Could you check a few things on this model? Use its own coordinates, in mm. Face numbers are marked on the shaded views. A direction names the side the tool comes from. Coordinates: 2 decimals unless noted, no trailing zeros. Order: outer loops, then holes, each group sorted by start corner. A loop starts at its lowest first (then second) coordinate and runs counter-clockwise, first axis right, second up.
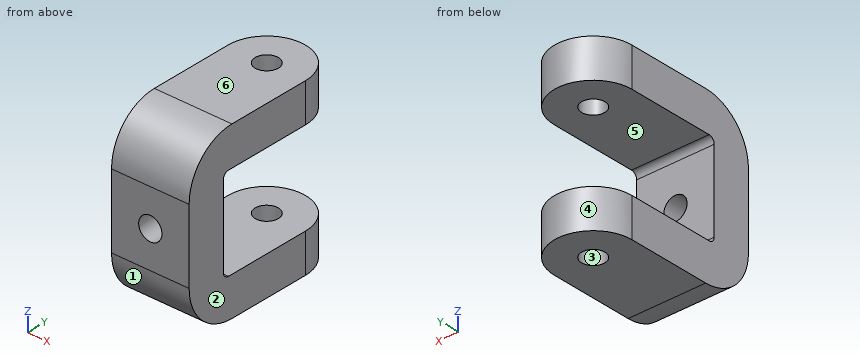
Autodesk Inventor part; units mm, degrees
ref_plane "YZ Plane" through (0, 0, 0) normal (1, 0, 0) x (0, 1, 0)
ref_plane "XZ Plane" through (0, 0, 0) normal (0, 1, 0) x (-1, 0, 0)
ref_plane "XY Plane" through (0, 0, 0) normal (0, 0, 1) x (1, 0, 0)
sketch "Sketch1" plane through (0, 0, 0) normal (0, 0, 1) x (1, 0, 0)
  arc A0 (5, 0) -> (-5, 0) centre (0, 0) ccw
  line L0 (-5, -17) -> (5, -17)
  line L1 (5, -17) -> (5, 0)
  line L2 (-5, -17) -> (-5, 0)
  circle A1 centre (0, 0) radius 1.5
  dimension "d0" = 3
  dimension "d1" = 5
  dimension "d2" = 17
extrude "Extrusion1" add sketch "Sketch1" along normal blind 22
sketch "Sketch2" plane through (5, -17, 0) normal (1, 0, 0) x (0, 0, -1)
  line L0 (0, 17) -> (0, 17)
  line L1 (0, 17) -> (-22, 17)
  line L2 (-22, 17) -> (-22, 17)
  line L3 (0, 17) -> (-22, 17)
  line L4 (0, 0) -> (0, 17)
  line L5 (0, 17) -> (-22, 17)
  line L6 (-22, 0) -> (-22, 17)
  line L7 (0, 0) -> (-22, 0)
  line L8 (-17, 5) -> (-5, 5)
  line L9 (-5, 5) -> (-5, 25)
  line L10 (-5, 25) -> (-17, 25)
  line L11 (-17, 25) -> (-17, 5)
  dimension "d5" = 5
  dimension "d6" = 5
  dimension "d7" = 5
  dimension "d8" = 20
extrude "Extrusion2" cut sketch "Sketch2" against normal blind 22 contours L9 L8 L11 L1 | L1 L11 L10 L9
sketch "Sketch3" plane through (-5, -17, 0) normal (0, -1, 0) x (1, 0, 0)
  line L0 (0, 0) -> (10, 0)
  line L1 (10, 0) -> (10, 22)
  line L2 (0, 22) -> (10, 22)
  line L3 (0, 0) -> (0, 22)
  circle A0 centre (5, 11) radius 1.5
  point P0 (5, 0)
  dimension "d11" = 22
  dimension "d12" = 10
  dimension "d13" = 3
  dimension "d14" = 5
  dimension "d15" = 11
extrude "Extrusion3" cut sketch "Sketch3" against normal blind 6 contours A0
fillet "Fillet1" radius 6.25 2 edges at (0, -17, 22) (0, -17, 0)
fillet "Fillet2" radius 0.75 2 edges at (0, -12, 17) (0, -12, 5)
equation "\"d14\" = 0.5 * d12"
equation "\"d15\" = 0.5 * d11"
properties part number "PulleyHolder"
Item 1: I need wall thicknesses on line 1 (X direction, y = 0, z = 3.25); line 2 (Z direction, x = 3.5, y = -0.5); line 3 (Z direction, x = 0, y = -15.5). Which ranges of each line are inside material? Lowest first, please.
Item 2: For pin 1 Ø1.8 at (x, z) = (0, 11) entering from +Y, with a flat end and sliding along its axis, tell me the tip position at first contact or that it passes through.
Item 3: Which directions (+Z, -Z, +X, -X, +Y, -Y) give clear straight access to the entire face, cutting with the end or side of a thin tool? Please do the marked faces 5 and 6.
Item 4: Thinking about a two-plate mould opening in Y: for the marked faces 1, 2, 3 and 4, which applies, +Y half, -Y half, draft (parallel to the pull), parting line (faces both ways), or undercut?
Item 5: Suppose I cut it at A-A (z = 11). List the corners of the cut face in (x, y) for me, and give its area (3 significant figures).
Item 6: Suppose I cut it at B-B (y = -5.25). List the corners of the cut face in (x, z) for me.
Item 7: Suppose I cut it at C-C (x = 0). List the corners of the cut face in (y, z) for me.
Item 8: Suppose I cut it at D-D (x = 3). List the corners of the cut face in (y, z) for me.
Geometry results:
1. line 1: x = -5 to -1.5, 1.5 to 5
1. line 2: z = 0 to 5, 17 to 22
1. line 3: z = 2.19 to 9.5, 12.5 to 19.81
2. pin 1: passes through
3. face 5: +X, -X, +Y
3. face 6: +Z, +X, -X, +Y, -Y
4. face 1: -Y half
4. face 2: draft
4. face 3: undercut
4. face 4: +Y half
5. outline: (-5, -17) - (-1.5, -17) - (-1.5, -12) - (-5, -12) - close; (1.5, -17) - (5, -17) - (5, -12) - (1.5, -12) - close
5. area: 35.0 mm2
6. outline: (-5, 0) - (5, 0) - (5, 5) - (-5, 5) - close; (-5, 17) - (5, 17) - (5, 22) - (-5, 22) - close
7. outline: (-17, 6.25) arc R6.25 ccw to (-10.75, 0) - (-1.5, 0) - (-1.5, 5) - (-11.25, 5) arc R0.75 cw to (-12, 5.75) - (-12, 9.5) - (-17, 9.5) - close; (-17, 12.5) - (-12, 12.5) - (-12, 16.25) arc R0.75 cw to (-11.25, 17) - (-1.5, 17) - (-1.5, 22) - (-10.75, 22) arc R6.25 ccw to (-17, 15.75) - close; (1.5, 0) - (5, 0) - (5, 5) - (1.5, 5) - close; (1.5, 17) - (5, 17) - (5, 22) - (1.5, 22) - close
8. outline: (-17, 6.25) arc R6.25 ccw to (-10.75, 0) - (4, 0) - (4, 5) - (-11.25, 5) arc R0.75 cw to (-12, 5.75) - (-12, 16.25) arc R0.75 cw to (-11.25, 17) - (4, 17) - (4, 22) - (-10.75, 22) arc R6.25 ccw to (-17, 15.75) - close
